For this review, take the finished solid that the model builds, in its own axes (mm). A direction names the side the tool comes from. Round coordinates to 2 decimals unless told otherwise and drop trailing zeros. Order: outer loops, then holes, each group sorted by start corner. A loop starts at its lowest first (then second) coordinate and runs counter-clockwise, first axis right, second up. Notation, with made-up numbers: (-28.75, -26) -> (-5.75, -26) arc R19 ccw to (-5.75, -13) -> close; hole circle Ø4 at (14, 76.25). An arc over 180 degrees is marked (long way). Put each result on its own line as item: value. Start each with the question number.
Autodesk Fusion 360 part; units mm, degrees
sketch "Skizze1" plane through (0, 0, 0) normal (0, 0, 1) x (1, 0, 0)
  line L0 (0, 0) -> (80, 0)
  line L1 (80, 0) -> (80, -40)
  line L2 (80, -40) -> (0, -40)
  line L3 (0, -40) -> (0, 0)
  line L4 (76, -36) -> (4, -36)
  line L5 (4, -36) -> (4, -4)
  line L6 (4, -4) -> (76, -4)
  line L7 (76, -4) -> (76, -36)
  dimension "d1" = 80
  dimension "d2" = 40
  dimension "d3" = 4
extrude "Extrusion1" add sketch "Skizze1" along normal blind 4 contours L4 L5 L6 L7
sketch "Skizze2" plane through (0, 0, 0) normal (0, 0, 1) x (1, 0, 0)
  line L0 (0, 0) -> (80, 0)
  line L1 (80, 0) -> (80, -40)
  line L2 (80, -40) -> (0, -40)
  line L3 (0, -40) -> (0, 0)
  line L4 (76, -4) -> (76, -36)
  line L5 (76, -36) -> (4, -36)
  line L6 (4, -36) -> (4, -4)
  line L7 (4, -4) -> (76, -4)
  dimension "d6" = 80
  dimension "d7" = 40
  dimension "d8" = 4
extrude "Extrusion2" add sketch "Skizze2" along normal blind 66
sketch "Skizze3" plane through (0, 0, 66) normal (0, 0, 1) x (-1, 0, 0)
  line L0 (-4, 36) -> (-4, 4)
  line L1 (-4, 4) -> (-76, 4)
  line L2 (-76, 4) -> (-76, 36)
  line L3 (-76, 36) -> (-4, 36)
  line L4 (0, 40) -> (-80, 40)
  line L5 (-80, 40) -> (-80, 0)
  line L6 (-80, 0) -> (0, 0)
  line L7 (0, 0) -> (0, 40)
  line L8 (-76, 9.9367) -> (-80, 9.9367)
  line L9 (-80, 9.9367) -> (-80, 29.9367)
  line L10 (-80, 29.9367) -> (-76, 29.9367)
  line L11 (-76, 29.9367) -> (-76, 9.9367)
  dimension "d11" = 4
  dimension "d12" = 20
extrude "Extrusion3" cut sketch "Skizze3" against normal blind 10 contours L2 L5 L8 L9 L10 L11
sketch "Skizze4" plane through (0, 0, 66) normal (0, 0, 1) x (-1, 0, 0)
  line L0 (-80, 29.9367) -> (-76, 29.9367)
  line L1 (-76, 29.9367) -> (-76, 36)
  line L2 (-76, 36) -> (-4, 36)
  line L3 (-4, 36) -> (-4, 4)
  line L4 (-4, 4) -> (-76, 4)
  line L5 (-76, 4) -> (-76, 9.9367)
  line L6 (-76, 9.9367) -> (-80, 9.9367)
  line L7 (-80, 9.9367) -> (-80, 0)
  line L8 (-80, 0) -> (0, 0)
  line L9 (0, 0) -> (0, 40)
  line L10 (0, 40) -> (-80, 40)
  line L11 (-80, 40) -> (-80, 29.9367)
  line L12 (-25, 0) -> (-51, 0)
  line L13 (-51, 0) -> (-51, 6)
  line L14 (-51, 6) -> (-25, 6)
  line L15 (-25, 6) -> (-25, 0)
  dimension "d15" = 26
extrude "Extrusion4" add sketch "Skizze4" along normal blind 3 contours L4 L8 L12 L13 L15 | L4 L13 L14 L15
sketch "Skizze5" plane through (0, 0, 66) normal (0, 0, 1) x (-1, 0, 0)
  line L0 (-25, 4) -> (-25, 0)
  line L1 (-25, 0) -> (0, 0)
  line L2 (0, 0) -> (0, 40)
  line L3 (0, 40) -> (-80, 40)
  line L4 (-80, 40) -> (-80, 29.9367)
  line L5 (-80, 29.9367) -> (-76, 29.9367)
  line L6 (-76, 29.9367) -> (-76, 36)
  line L7 (-76, 36) -> (-4, 36)
  line L8 (-4, 36) -> (-4, 4)
  line L9 (-4, 4) -> (-25, 4)
  line L10 (-25, 40) -> (-50, 40)
  line L11 (-50, 40) -> (-50, 34)
  line L12 (-50, 34) -> (-25, 34)
  line L13 (-25, 34) -> (-25, 40)
  dimension "d18" = 25
  dimension "d19" = 6
extrude "Extrusion5" add sketch "Skizze5" along normal blind 3 contours L7 L11 L12 L13 | L3 L7 L10 L11 L13
fillet "Abrundung1" radius 1 18 edges at (38, -6, 69) (51, -6, 67.5) (25, -6, 67.5) (38, -6, 66) (51, -3, 69) (37.5, -40, 69) (50, -37, 69) (50, -34, 67.5) (37.5, -34, 69) (25, -37, 69) (25, -3, 69) (25, -34, 67.5) (37.5, -34, 66) (25, -35, 66) (51, -5, 66) (50, -35, 66) (25, -5, 66) (38, 0, 69)
Item 1: Mouldability with a two-part tool opening along X and no side actions: class faces 5 (the face through (38, -3, 69)), 6 (the face through (39, -4, 35)), 7 (the face through (50, -38, 67)) as +X half, -X half, draft (parallel to the pull), parting line (faces both ways), or undercut.
Item 2: For L1, parallel to X at y = -15.5, z = 13.5; L2, parallel to Y at x = 55.5, z = 6.5; L3, parallel to Z at x = 31, y = -4.5, list the stretches that pass through material, from the lowest coordinate up.
Item 3: Insertion check: pin 1 Ø11 at (x, y) = (72.5, -7) entering from +Z; pin 2 Ø2 at (y, z) = (-37, 67.5) entering from +X; pin 3 Ø0.6 at (y, z) = (-37, 67) entering from -X. Each pin has a flat end and moves straight along its axis. Give the tip position at first contact, or say it passes through.
Item 4: Consider section A-A, the plane z = 36.5. Write out the cut boundary in (x, y), plus the area to 3 significant figures.
Item 5: Consider section D-D, the plane x = 40.5. Write out the cut boundary in (y, z).
Item 6: Consider section B-B, the plane y = -17. Write out the cut boundary in (x, z).
Item 7: Tool access review of faces 1 (the face through (4, -20, 35)), 2 (the face through (78, -20, 56)), 3 (the face through (65, -3, 66)), 4 (the face through (25, -3, 67)): name each direction out of +Z, -Z, +X, -X, +Y, -Y from which nothing blocks a thin tool from reaching the whole face with its end or side.
Item 8: Consider section C-C, the plane x = 7.5. Write out the cut boundary in (y, z), plus the area to 3 significant figures.
Evaluation:
1. face 5: draft
1. face 6: undercut
1. face 7: +X half
2. L1: x = 0 to 4, 76 to 80
2. L2: y = -40 to -36, -4 to 0
2. L3: z = 0 to 4, 66 to 69
3. pin 1: stops at z = 66
3. pin 2: stops at x = 50
3. pin 3: stops at x = 25
4. outline: (0, -40) -> (80, -40) -> (80, 0) -> (0, 0) -> close; hole (4, -36) -> (76, -36) -> (76, -4) -> (4, -4) -> close
4. area: 896 mm^2
5. outline: (-40, 0) -> (0, 0) -> (0, 68) arc R1 ccw to (-1, 69) -> (-5, 69) arc R1 ccw to (-6, 68) -> (-6, 67) arc R1 ccw to (-5, 66) -> (-4, 66) -> (-4, 4) -> (-36, 4) -> (-36, 66) -> (-35, 66) arc R1 ccw to (-34, 67) -> (-34, 68) arc R1 ccw to (-35, 69) -> (-39, 69) arc R1 ccw to (-40, 68) -> close
6. outline: (0, 0) -> (80, 0) -> (80, 56) -> (76, 56) -> (76, 4) -> (4, 4) -> (4, 66) -> (0, 66) -> close
7. face 1: +Z
7. face 2: +Z, +X
7. face 3: +Z, +X, +Y, -Y
7. face 4: +Z, -X, +Y, -Y
8. outline: (-40, 0) -> (0, 0) -> (0, 66) -> (-4, 66) -> (-4, 4) -> (-36, 4) -> (-36, 66) -> (-40, 66) -> close
8. area: 656 mm^2
